Can you work these out from the model? Positions are in its coordinate system, mm. Coordinates: 2 decimals unless noted, no trailing zeros. Order: outer loops, then holes, each group sorted by start corner. A loop starts at its lowest first (then second) coordinate and runs counter-clockwise, first axis right, second up. Notation, with made-up numbers: (24, 46.5) -> (44, 46.5) arc R31 cw to (44, 77.5) -> close; hole circle Ø3 at (-16, 83.5). An arc over 180 degrees is marked (long way). Use a Markdown table: item, result. Add a question column.
1. For pin 1 Ø1 at (x, y) = (2, -2) entering from -Z; pin 2 Ø1.7 at (x, z) = (0.5, 4) entering from +Y; pin 3 Ø1 at (y, z) = (2.5, 147.5) entering from -X, each with a flat end and sliding along its axis, tell me the tip position at first contact or that it passes through.
2. Suppose I cut it at A-A, the plane z = 45. List the corners of the cut face in (x, y) for me (3 decimals).
3. If I drill on line 1 along X through (y, z) = (-0.2, 3.81); line 2 along X through (y, z) = (-1.45, 3.81); line 3 along Z through (x, y) = (0, 0.05), over which ranges is the centre line in solid material (lowest first)? Write a range as from..to.
4. Suppose I cut it at B-B, the plane z = 86. List the corners of the cut face in (x, y) for me (3 decimals), then the cut area to 3 significant figures.
Autodesk Inventor part; units mm, degrees
ref_plane "YZ Plane" through (0, 0, 0) normal (1, 0, 0) x (0, 1, 0)
ref_plane "XZ Plane" through (0, 0, 0) normal (0, 1, 0) x (-1, 0, 0)
ref_plane "XY Plane" through (0, 0, 0) normal (0, 0, 1) x (1, 0, 0)
sketch "Sketch1" plane through (0, 0, 0) normal (0, 0, 1) x (1, 0, 0)
  circle A0 centre (0, 0) radius 3.175
  dimension "d0" = 6.35
extrude "Extrusion1" add sketch "Sketch1" along normal blind 177.8
sketch "Sketch2" plane through (0, 0, 0) normal (0, 0, 1) x (1, 0, 0)
  circle A0 centre (0, 0) radius 3.175
  line L0 (2.5773, 1.8542) -> (-2.5773, 1.8542)
  line L1 (0, 4.445) -> (0, -4.445)
  line L2 (-4.445, 0) -> (4.445, 0)
  line L3 (2.8511, 1.397) -> (-2.8511, 1.397)
  line L4 (2.1082, 1.397) -> (2.4308, 0.8382)
  line L5 (2.4308, 0.8382) -> (-2.4308, 0.8382)
  line L6 (-2.4308, 0.8382) -> (-2.1082, 1.397)
  line L7 (0, 0) -> (0, 3.175)
  dimension "d6" = 1.397
  dimension "d9" = 60
  dimension "d10" = 4.2164
  dimension "d11" = 0.5588
  dimension "d40" = 0.4572
extrude "Extrusion3" cut sketch "Sketch2" along normal blind 12.7 contours L3 L1 L0 A0 | L1 L3 A0 L0
extrude "Extrusion4" cut sketch "Sketch2" along normal up to surface (12.7 mm away) contours L4 L5 L1 L3 | L5 L6 L3 L1
sketch "Sketch3" plane through (-2.4308, 0.8382, 12.7) normal (0, 1, 0) x (1, 0, 0)
  line L0 (0, 12.7) -> (4.8616, 12.7)
  line L1 (2.4308, 48.26) -> (2.4308, -200.66)
  point P0 (2.4308, 12.7)
  point P1 (2.4308, 8.89)
  dimension "d14" = 3.81
hole "Hole1" at (0, 0.8382, 3.81) direction (0, -1, 0) diameter 2.0066 end through all
sketch "Sketch4" plane through (0, 0, 0) normal (1, 0, 0) x (0, 1, 0)
  line L0 (0, 213.36) -> (0, -35.56)
  line L1 (-3.175, 0) -> (-3.175, 177.8)
  line L2 (0, 0) -> (-3.175, 5.4993)
  line L3 (-3.175, 5.4993) -> (-3.175, 0)
  line L4 (-3.175, 0) -> (0, 0)
  dimension "d23" = 30
extrude "Extrusion5" cut sketch "Sketch4" along normal mid plane 12.7
chamfer "Chamfer1" distance 0.254 distance2 0.381 1 edges at (-2.2695, 1.1176, 0) measured on face at (0.8103, 0.2794, 0)
chamfer "Chamfer2" distance 0.254 distance2 0.381 1 edges at (2.2695, 1.1176, 0) measured on face at (0.8103, 0.2794, 0)
chamfer "Chamfer3" distance 0.762 angle 45 1 edges at (-3.175, 0, 177.8)
extrude "Extrusion7" cut sketch "Sketch2" along normal blind 50.8 contours L3 L1 L0 A0 | L0 L1 A0 | L1 L0 A0 | L1 L3 A0 L0
sketch "Sketch6" plane through (-2.1082, 1.397, 12.7) normal (0, 1, 0) x (1, 0, 0)
  line L0 (-0.7429, -38.1) -> (4.9593, -38.1)
  line L1 (0, 0) -> (4.2164, 0)
  line L2 (2.1082, 48.26) -> (2.1082, -200.66)
  line L3 (8.3312, 12.7) -> (-4.1148, 12.7)
  line L4 (6.5532, -1.27) -> (-2.3368, -1.27)
  line L5 (-2.3368, -1.27) -> (-2.3368, -38.1)
  line L6 (-2.3368, -38.1) -> (6.5532, -38.1)
  line L7 (6.5532, -38.1) -> (6.5532, -1.27)
  line L8 (6.5532, -1.27) -> (-2.3368, -38.1) construction
  line L9 (-2.3368, -1.27) -> (6.5532, -38.1) construction
  point P0 (2.1082, 12.7)
  point P1 (2.1082, -19.685)
  dimension "d43" = 0
  dimension "d44" = 1.27
  dimension "d45" = 8.89
extrude "Extrusion8" cut sketch "Sketch6" against normal blind 0.508
sketch "Sketch8" plane through (-2.8511, 1.397, 13.97) normal (0, 1, 0) x (1, 0, 0)
  point P0 (2.8511, 13.97)
sketch "Sketch9" plane through (-2.1082, 1.397, 12.7) normal (0, 1, 0) x (1, 0, 0)
  point P0 (2.1082, 12.7)
sketch "Sketch10" plane through (-2.1082, 1.397, 12.7) normal (0, 1, 0) x (1, 0, 0)
  point P0 (2.1082, 12.7)
fillet "Fillet3" radius 1.016 2 edges at (-2.2695, 1.1176, 12.7) (2.2695, 1.1176, 12.7)
sketch "Sketch11" plane through (0, 0, 0) normal (1, 0, 0) x (0, 1, 0)
  line L0 (0.889, 13.97) -> (0.889, 50.8)
  line L1 (3.175, 50.8) -> (3.175, 177.038)
  line L2 (1.016, 50.8) -> (3.175, 54.5395)
  line L3 (0.889, 13.97) -> (1.397, 13.97)
  line L4 (-4.445, 0) -> (4.445, 0)
  line L5 (1.016, 13.97) -> (1.397, 13.3101)
  line L6 (1.397, 13.3101) -> (1.397, 13.97)
  line L7 (1.016, 13.97) -> (1.397, 13.97)
  line L8 (0.8382, 12.7) -> (1.397, 12.7)
  line L9 (3.175, 54.5395) -> (3.175, 50.8)
  line L10 (3.175, 50.8) -> (0.889, 50.8)
  line L11 (1.016, 50.8) -> (3.175, 50.8)
  point P0 (0, 0)
  dimension "d56" = 0.127
  dimension "d57" = 13.97
  dimension "d58" = 0.127
  dimension "d59" = 30
  dimension "d60" = 0.6101
extrude "Extrusion10" cut sketch "Sketch11" along normal mid plane 6.35
properties part number "J007778" material "ALUMINUM, 6061-T651"
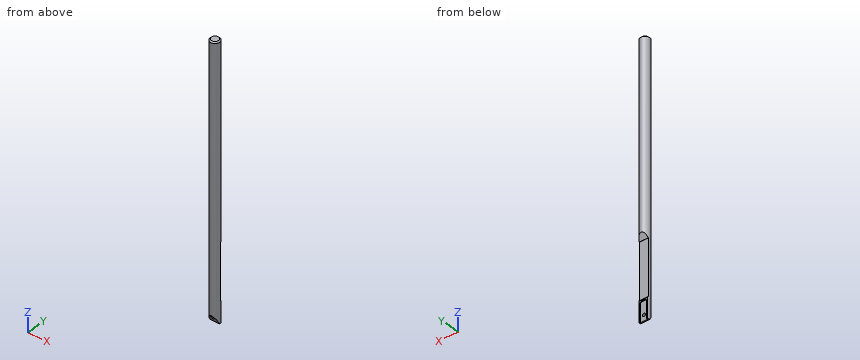
Worked out:
| question | item | result |
|---|---|---|
| 1 | pin 1 | stops at z = 2.6 |
| 1 | pin 2 | stops at y = 0.84 |
| 1 | pin 3 | stops at x = -2.47 |
| 2 | outline | (-3.048, 0.889) arc R3.175 ccw (long way) to (3.048, 0.889) -> close |
| 3 | line 1 | x = -3.17..-1, 1..3.17 |
| 3 | line 2 | x = -2.82..-1, 1..2.82 |
| 3 | line 3 | z = 0..2.81, 4.81..177.8 |
| 4 | outline | circle Ø6.35 at (0, 0) |
| 4 | area | 31.7 mm² |
